Print and shaded views of the part. All mm, measured from the part's lowest x, y and z. A direction names the side the tool comes from. Round coordinates to 2 decimals unless told otherwise and drop trailing zeros. Write each loop counter-clockwise with the first axis right and the second up, starting at its lowest first coordinate (ties: lowest second). Pieces come first, ordered by that corner, then holes. Notation, with made-up numbers: (-27.5, -8) -> (-17.5, -8) arc R26 ccw to (-17.5, 17) -> close; hole circle Ø7 at (26, -21.5). An arc over 180 degrees is marked (long way). Return JSON: item names as keys, results as strings. Group by question number.
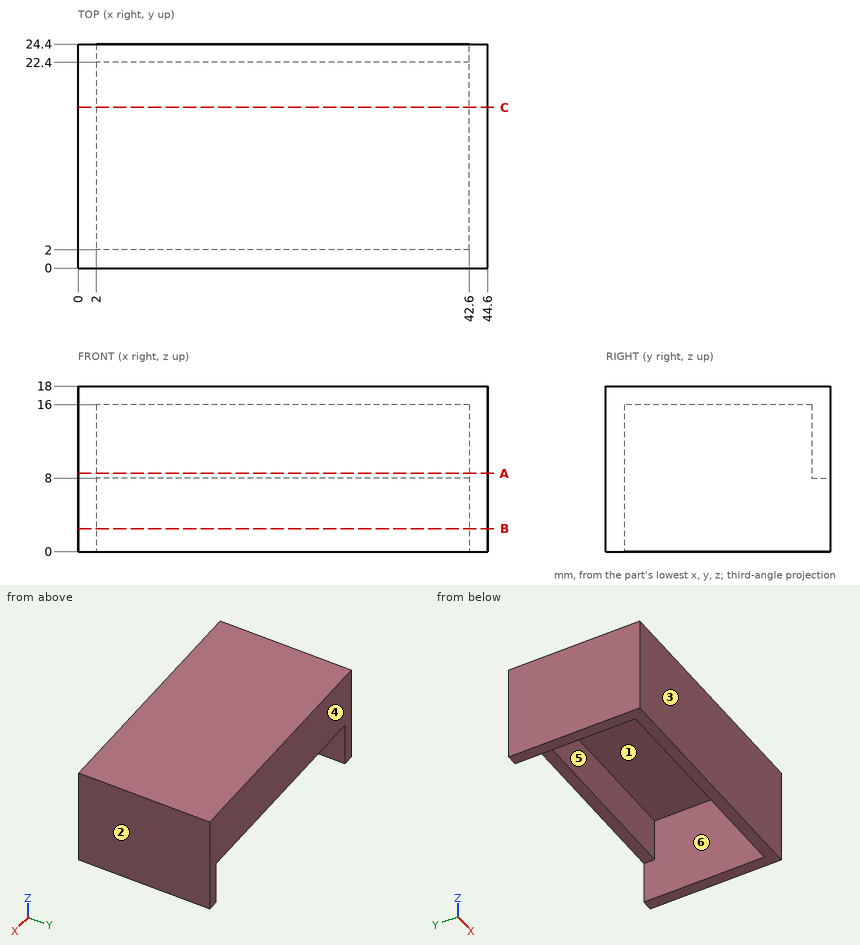
Item 1: Two-plate mould, pull along Y, no slides. Class the marked faces 3, 4, 5 and 6: released by +Y, released by -Y, zero draft, split by the parting line, or undercut.
Item 2: Wall check: L1, parallel to Y at x = 7, z = 10.5; L2, parallel to X at y = 18.25, z = 4.75; L3, parallel to Y at x = 30, z = 6.5. Give the ranges that are in metal, low to high.
Item 3: Flat gauge pins, fed straight in: P1, Ø6, axis at x = 24.5, y = 7, coming from the -Z side; P2, Ø1, axis at x = 32, y = 23, coming from the -Z side. Where does each tip first touch, or does it go through?
Item 4: Cut at C-C (y = 17.5). Write the cut outline in (x, z), then the cut area to 3 significant figures.
Item 5: Cut at A-A (z = 8.5). Write the cut outline in (x, y).
Item 6: Which spindle directions (+Z, -Z, +X, -X, +Y, -Y) get a long thin tool onto all of the face, cutting with end or side? Do the marked faces 1 and 2. Say none if no direction does.
Item 7: Cut at B-B (z = 2.5). Write the cut outline in (x, y).
Checks:
{
 "1": {"face 3": "released by -Y", "face 4": "released by +Y", "face 5": "undercut", "face 6": "undercut"},
 "2": {"L1": "y = 0 to 2, 22.4 to 24.4", "L2": "x = 0 to 2, 42.6 to 44.6", "L3": "y = 0 to 2"},
 "3": {"P1": "stops at z = 16", "P2": "stops at z = 8"},
 "4": {"outline": "(0, 0) -> (2, 0) -> (2, 16) -> (42.6, 16) -> (42.6, 0) -> (44.6, 0) -> (44.6, 18) -> (0, 18) -> close", "area": "153 mm2"},
 "5": {"outline": "(0, 0) -> (44.6, 0) -> (44.6, 24.4) -> (0, 24.4) -> close; hole (2, 2) -> (42.6, 2) -> (42.6, 22.4) -> (2, 22.4) -> close"},
 "6": {"face 1": "-Z", "face 2": "+Z, -Z, +X, +Y, -Y"},
 "7": {"outline": "(0, 0) -> (44.6, 0) -> (44.6, 24.4) -> (42.6, 24.4) -> (42.6, 2) -> (2, 2) -> (2, 24.4) -> (0, 24.4) -> close"}
}
